from build123d import *

# Parameters (mm, degrees)
SKETCH2_W           = 19.05
SKETCH2_H           = 37.278922504
BOSS_EXTRUDE1_DEPTH = 428.225
BOSS_EXTRUDE2_DEPTH = 356
SKETCH6_R           = 3.3655
CUT_EXTRUDE1_DEPTH  = 25.4


with BuildPart() as part:
    # Sketch2 → Boss-Extrude1 (new body)
    with BuildSketch(Plane.ZY.offset(11.1125)):
        with Locations((9.525, 246.563328153)):
            Rectangle(SKETCH2_W, SKETCH2_H)
    extrude(amount=-BOSS_EXTRUDE1_DEPTH)

    # Sketch5 → Boss-Extrude2 (add)
    with BuildSketch(Plane.ZY.offset(-381)):
        Polygon((19.05, 227.923866901), (0, 227.923866901), (0, 201.997670401), (19.05, 224.857670401), align=None)
        Polygon((19.05, 224.857670401), (0, 201.997670401), (0, 192.286298431), (19.05, 215.146298431), align=None)
        Polygon((19.05, 215.146298431), (0, 192.286298431), (0, 166.012618521), (19.05, 188.872618521), align=None)
        Polygon((0, 166.012618521), (19.05, 166.012618521), (19.05, 188.872618521), align=None)
    extrude(amount=BOSS_EXTRUDE2_DEPTH)

    # Sketch6 → Cut-Extrude1 (cut)
    with BuildSketch(Plane(origin=(203, 213.395866862, -1.905), x_dir=(-1, 0, 0), z_dir=(0, 0, -1))):
        with Locations(Location((192.0145, 34.026922543, 0), (0, 0, 90))):
            Circle(SKETCH6_R)
    cut_extrude1 = extrude(amount=-CUT_EXTRUDE1_DEPTH, mode=Mode.SUBTRACT)

    # Mirror1: Cut-Extrude1 across plane
    add(cut_extrude1.mirror(Plane.ZY.offset(-203)), mode=Mode.SUBTRACT)


solid = part.part
Can you work these out from the model? Positions are in its coordinate system, mm. A direction names the side the tool comes from. Round coordinates to 2 decimals unless told otherwise and drop trailing zeros. Write each loop counter-clockwise with the first axis right and the second up, starting at its lowest first coordinate (ties: lowest second). Pieces come first, ordered by that corner, then holes. Notation, with made-up numbers: (-31, 43.5) -> (-18, 43.5) arc R16 ccw to (-18, 51.5) -> close; hole circle Ø9 at (29, 29). An arc over 180 degrees is marked (long way). One line per question, with ' | ' between items. Start each with the question number.
1) On a 3-axis mill with a long thin cutter (end or side, diameter ignored), from which of +Z, -Z, +X, -X, +Y, -Y can I reach the whole of each face in a straight line? I mean faces 4 (the flat face through (200, 215, 0)), 5 (the flat face through (25, 197, 9)), 6 (the flat face through (399, 227.924, 9)). Say none if no direction works.
2) Suppose I cut it at C-C on y = 222. Write out the boundary of the cut face in (x, z), then the cut area to 3 significant figures.
3) Suppose I cut it at A-A on z = 4. Write out the boundary of the cut face in (x, y).
4) I need wall thicknesses on line 1 (X direction, y = 213.5, z = 3.75); line 2 (Y direction, x = 15.5, z = 8.75); line 3 (Y direction, x = 392, z = 10.75). Which ranges of each line are inside material? Lowest first, please. Write a range as [from, to].
5) Suppose I cut it at B-B on x = 18. Write out the boundary of the cut face in (y, z), then the cut area to 3 significant figures.
6) I'm going to push flat-ended pins straight in: P1, Ø5.5, axis at x = 402, z = 13.5, coming from the -Y side; P2, Ø5.5, axis at y = 206, z = 8, coming from the +X side. Where does each tip first touch, or does it pass through?
7) If we mould it in two halves opening along Y, with no side actions, what happens to faces 1 (the flat face through (205, 166.013, 9)), 2 (the cylindrical face through (391.68, 246.98, 9.39)), 3 (the flat face through (381, 197, 9))? For each: released by +Y, released by -Y, zero draft, split by the parting line, or undercut.
Return value:
1) face 4: -Z, +X, -X, +Y, -Y | face 5: +Z, -Z, -X, -Y | face 6: +Z, -Z, +X, -Y
2) outline: (25, 0) -> (381, 0) -> (381, 19.05) -> (25, 19.05) -> close | area: 6,780 mm2
3) outline: (-11.11, 227.92) -> (25, 227.92) -> (25, 166.01) -> (381, 166.01) -> (381, 227.92) -> (417.11, 227.92) -> (417.11, 265.2) -> (-11.11, 265.2) -> close; hole circle Ø6.73 at (10.99, 247.42); hole circle Ø6.73 at (395.01, 247.42)
4) line 1: x = [25, 381] | line 2: y = [227.92, 265.2] | line 3: y = [227.92, 245.93], [248.92, 265.2]
5) outline: (227.92, 0) -> (265.2, 0) -> (265.2, 19.05) -> (227.92, 19.05) -> close | area: 710 mm2
6) P1: stops at y = 227.92 | P2: stops at x = 381
7) face 1: released by -Y | face 2: undercut | face 3: zero draft
